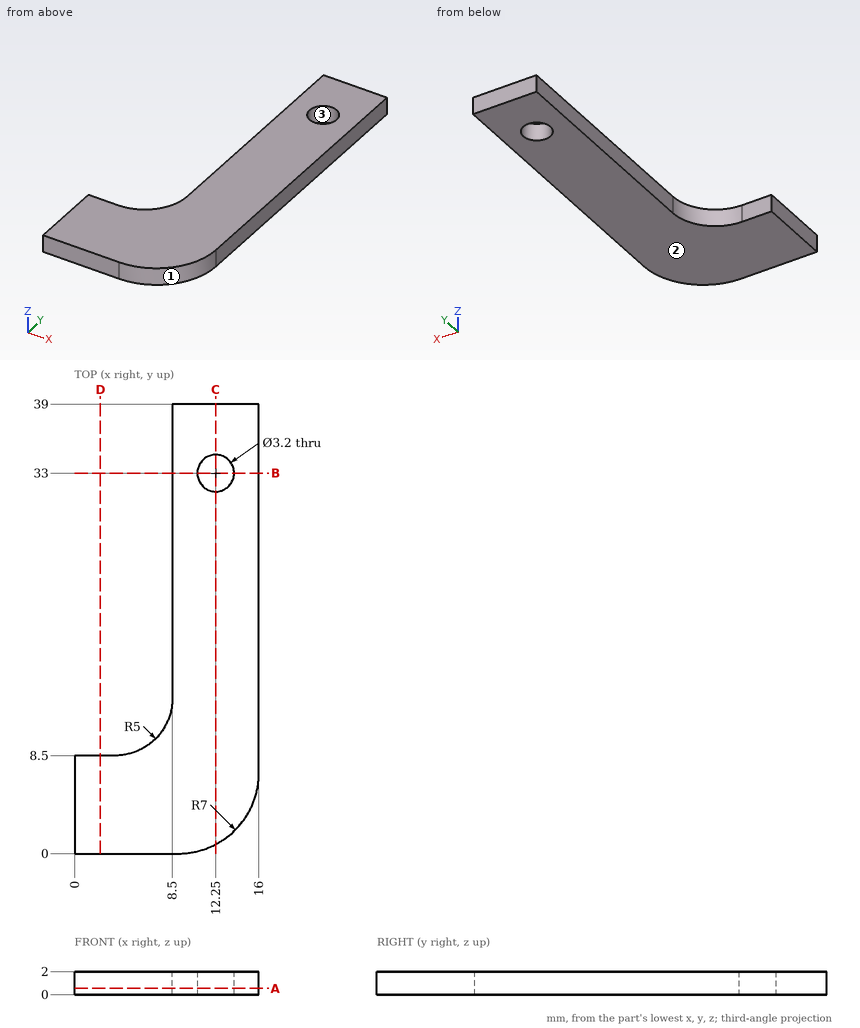
Geometry check sheet. Reference: drawing and pictorial views, mm from the part's lowest x, y, z. Give positions to 0.01 mm unless a question says otherwise; leave off trailing zeros. Write each loop counter-clockwise with the first axis right and the second up, starting at its lowest first coordinate (ties: lowest second). Pieces come first, ordered by that corner, then holes. Notation, with made-up numbers: M 88.25,81.25 L 145.25,81.25 A19 ccw 145.25,85.25 Z; hole C 79,-16 d10. An arc over 180 degrees is marked long. Put each result on its own line as item: value. Start each with the question number.
1. Scan lines: line 1 along X through (y, z) = (36.5, 0.5); line 2 along Y through (x, z) = (12.25, 1.3); line 3 along X through (y, z) = (4.5, 1.65). Record each from-to range of solid material in increasing order. Write a range as [from, to].
2. Section check C-C (x = 12.25). Record the cut outline in (y, z), and give its area (3 significant figures).
3. Draft check along Y on the marked faces 1, 2 and 3. Enter one of: +Y half, -Y half, draft (parallel to the pull), parting line (faces both ways), or undercut.
4. Section check B-B (y = 33). Record the cut outline in (x, z), and give its area (3 significant figures).
5. Section check D-D (x = 2.25). Record the cut outline in (y, z), and give its area (3 significant figures).
6. Section check A-A (z = 0.55). Record the cut outline in (x, y), and give its area (3 significant figures).
7. Go/stop test with flat-tipped pins: pin 1 Ø1 at (y, z) = (21, 1) entering from -X; pin 2 Ø0.6 at (x, z) = (1.5, 1.5) entering from +Y. Record where each tip stops, or that it passes through.
Answer list:
1. line 1: [8.5, 16]
1. line 2: [0.8, 31.4], [34.6, 39]
1. line 3: [0, 15.54]
2. outline: M 0.8,0 L 31.4,0 L 31.4,2 L 0.8,2 Z; M 34.6,0 L 39,0 L 39,2 L 34.6,2 Z
2. area: 70.0 mm2
3. face 1: -Y half
3. face 2: draft
3. face 3: undercut
4. outline: M 8.5,0 L 10.65,0 L 10.65,2 L 8.5,2 Z; M 13.85,0 L 16,0 L 16,2 L 13.85,2 Z
4. area: 8.60 mm2
5. outline: M 0,0 L 8.5,0 L 8.5,2 L 0,2 Z
5. area: 17.0 mm2
6. outline: M 0,0 L 9,0 A7 ccw 16,7 L 16,39 L 8.5,39 L 8.5,13.5 A5 cw 3.5,8.5 L 0,8.5 Z; hole C 12.25,33 d3.2
6. area: 352 mm2
7. pin 1: x = 8.5
7. pin 2: y = 8.5
